Could you check a few things on this model? Use its own coordinates, in mm. Face numbers are marked on the shaded views. A direction names the side the tool comes from. Round coordinates to 2 decimals unless told otherwise and drop trailing zeros. Answer in a Markdown table with one row per item.
from build123d import *

# Parameters (mm, degrees)
CROQUIS2_W            = 19
CROQUIS2_H            = 7
CROQUIS1_W            = 22
CROQUIS1_H            = 10
CORTAR_EXTRUIR1_REACH = 5.2
CROQUIS1_3_W          = 17
CROQUIS1_3_H          = 5
CORTAR_EXTRUIR2_REACH = 7


with BuildPart() as part:
    # Croquis2 → Recubrir1 section 0
    with BuildSketch(Plane(origin=(0, 3.2, 0), x_dir=(1, 0, 0), z_dir=(0, 1, 0))):
        Rectangle(CROQUIS2_W, CROQUIS2_H)
    # Croquis1 → Recubrir1 section 1
    with BuildSketch(Plane(origin=(0, 0, 0), x_dir=(1, 0, 0), z_dir=(0, 1, 0))):
        Rectangle(CROQUIS1_W, CROQUIS1_H)
    loft()

    # Croquis1<3> → Cortar-Extruir1 (cut, up to next)
    with BuildSketch(Plane(origin=(0, 0, 0), x_dir=(1, 0, 0), z_dir=(0, 1, 0)), mode=Mode.PRIVATE) as cortar_extruir1_sk1:
        Rectangle(CROQUIS1_3_W, CROQUIS1_3_H)
    cortar_extruir1_tool1 = extrude(cortar_extruir1_sk1.sketch, amount=CORTAR_EXTRUIR1_REACH, mode=Mode.PRIVATE) & part.part
    add(cortar_extruir1_tool1.solids().sort_by_distance((0, 0, 0))[0], mode=Mode.SUBTRACT)

    # Croquis4 → Cortar-Extruir2 (cut, up to next)
    with BuildSketch(Plane.XY, mode=Mode.PRIVATE) as cortar_extruir2_sk1:
        Polygon((7.216878365, 1.5), (14.43375673, 14), (7.216878365, 26.5), (-7.216878365, 26.5), (-14.43375673, 14), (-7.216878365, 1.5), align=None)
    cortar_extruir2_tool1 = extrude(cortar_extruir2_sk1.sketch, amount=-CORTAR_EXTRUIR2_REACH, mode=Mode.PRIVATE) & part.part
    add(cortar_extruir2_tool1.solids().sort_by_distance((0, 14, 0))[0], mode=Mode.SUBTRACT)


solid = part.part
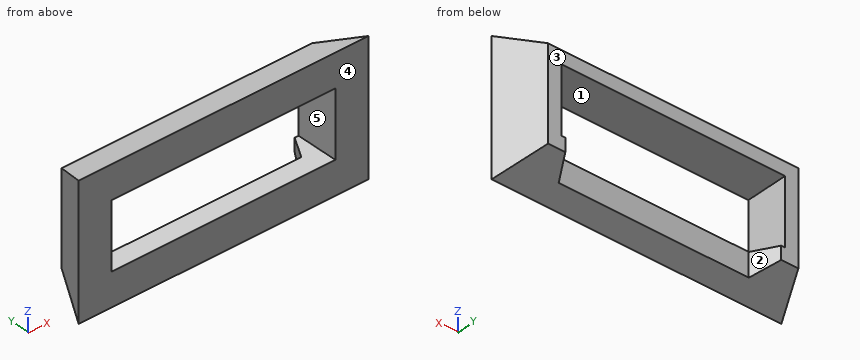
1) Thinking about a two-plate mould opening in Z: for the marked faces 4 and 5, which applies, +Z half, -Z half, draft (parallel to the pull), parting line (faces both ways), or undercut?
Findings:
| item | result |
|---|---|
| face 4 | draft |
| face 5 | undercut |
2) For the marked faces 1, 2 and 3, which set-ups out of +Z, -Z, +X, -X, +Y, -Y let a thin tool reach every point of the face, with its end or its side?
Findings:
| item | result |
|---|---|
| face 1 | +Y, -Y |
| face 2 | -Z, +Y |
| face 3 | +Z, -Z, +X, -X, +Y |
3) For pin 1 (3 mm diameter, centred on x = -4.5, z = 2.5, fed in from -Y); pin 2 (1.4 mm diameter, centred on x = 0, z = -4, fed in from +Y); pin 3 (1 mm diameter, centred on y = 2, z = -1, fed in from -X); pin 4 (1.6 mm diameter, centred on y = 2, z = 0, fed in from +X), each with a flat end and sliding along its axis, tell me the tip position at first contact or that it passes through.
Findings:
| item | result |
|---|---|
| pin 1 | stops at y = 0 |
| pin 2 | stops at y = 1.5 |
| pin 3 | stops at x = -10.3 |
| pin 4 | stops at x = 10.44 |
4) Please list where these lines run through material, in increasing order: line 1 (Y direction, x = -2, z = -3); line 2 (Z direction, x = 5.5, y = 0.85); line 3 (X direction, y = 2.6, z = 1).
Findings:
| item | result |
|---|---|
| line 1 | y = 0 to 1.5 |
| line 2 | z = -4.6 to -2.5, 2.5 to 4.6 |
| line 3 | x = -9.78 to -8.5, 8.5 to 9.78 |
